Read the model definition and answer for the solid it produces. Units are mm, in the model's axes. Face numbers are marked on the shaded views. Give positions to 0.01 mm unless a question says otherwise; leave off trailing zeros. Write each loop counter-clockwise with the first axis right and the second up, starting at its lowest first coordinate (ties: lowest second). Pieces come first, ordered by that corner, then holes. Notation, with made-up numbers: M -3.5,28 L 49.5,28 A10 cw 49.5,44 Z; hole C 38,41.5 d2. An arc over 180 degrees is marked long. Put each result on its own line as item: value.
from build123d import *

# Parameters (mm, degrees)
SKETCH1_R               = 16.8275
SKETCH1_R_2             = 12.7
BOSS_EXTRUDE1_DEPTH     = 304.8
CUT_EXTRUDE1_DEPTH      = 306.727606723
CUT_EXTRUDE1_DEPTH_BACK = 306.727606723
SKETCH2_R               = 2.2479
CUT_EXTRUDE2_DEPTH      = 306.727606834
CUT_EXTRUDE2_DEPTH_BACK = 306.727606834
SKETCH3_R               = 2.2479


with BuildPart() as part:
    # Sketch1 → Boss-Extrude1 (new body)
    with BuildSketch(Plane(origin=(0, 0, 0), x_dir=(1, 0, 0), z_dir=(0, 1, 0))):
        with Locations(Location((0, 0, 0), (0, 0, 90))):
            Circle(SKETCH1_R)
        with Locations(Location((0, 0, 0), (0, 0, 90))):
            Circle(SKETCH1_R_2, mode=Mode.SUBTRACT)
    extrude(amount=BOSS_EXTRUDE1_DEPTH)

    # Sketch2 → Cut-Extrude1 (cut, two sides: drawn at the far end of the back side and taken through both)
    with BuildSketch(Plane.XY.offset(-CUT_EXTRUDE1_DEPTH_BACK)):
        with Locations((0, 203.2)):
            Circle(SKETCH2_R)
    extrude(amount=CUT_EXTRUDE1_DEPTH + CUT_EXTRUDE1_DEPTH_BACK, mode=Mode.SUBTRACT)

    # Sketch3 → Cut-Extrude2 (cut, two sides: drawn at the far end of the back side and taken through both)
    with BuildSketch(Plane(origin=(0, 0, 0), x_dir=(0, 0, -1), z_dir=(1, 0, 0)).offset(-CUT_EXTRUDE2_DEPTH_BACK)):
        with Locations((0, 6.35)):
            Circle(SKETCH3_R)
    extrude(amount=CUT_EXTRUDE2_DEPTH + CUT_EXTRUDE2_DEPTH_BACK, mode=Mode.SUBTRACT)


solid = part.part
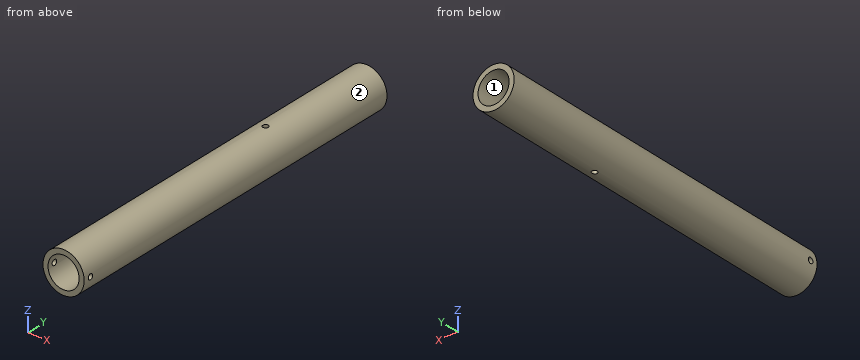
(1) Given pin 1 Ø7 at (y, z) = (6.35, 0) entering from +X; pin 2 Ø8 at (x, y) = (-9, 40) entering from +Z; pin 3 Ø5 at (y, z) = (37, -7.5) entering from +X; pin 4 Ø3 at (y, z) = (74.5, -11) entering from -X, each flat-ended and moving along its own axis, determine where each tip first touches the part or whether it passes through.
Result:
pin 1: stops at x = 16.83
pin 2: stops at z = 16.07
pin 3: stops at x = 16.07
pin 4: stops at x = -13.89
(2) Section C-C on y = 123.5 is taken. Determine the outline of the cut face in (x, z) (1 decimal), and give its area (3 significant figures).
Result:
outline: C 0,0 d33.7; hole C 0,0 d25.4
area: 383 mm²
(3) Section A-A on z = -5 is taken. Determine the outline of the cut face in (x, y).
Result:
outline: M -16.07,0 L -11.67,0 L -11.67,304.8 L -16.07,304.8 Z; M 11.67,0 L 16.07,0 L 16.07,304.8 L 11.67,304.8 Z
(4) Section B-B on x = 9 is taken. Determine the outline of the cut face in (y, z).
Result:
outline: M 0,-14.22 L 304.8,-14.22 L 304.8,-8.96 L 0,-8.96 Z; M 0,8.96 L 304.8,8.96 L 304.8,14.22 L 0,14.22 Z
(5) Straight lines are drawn through the part: line 1 along Y through (x, z) = (14, 0); line 2 along Z through (x, y) = (-1, 153); line 3 along Z through (x, y) = (-10, 145). For each, find the intervals that lie inside material, in ascending order. Write a range as from..to.
Result:
line 1: y = 0..4.1, 8.6..304.8
line 2: z = -16.8..-12.66, 12.66..16.8
line 3: z = -13.53..-7.83, 7.83..13.53
(6) For a pull along X with two mould halves and no side action, classify the marked faces 1 and 2 as +X half, -X half, draft (parallel to the pull), parting line (faces both ways), or undercut.
Result:
face 1: undercut
face 2: parting line
